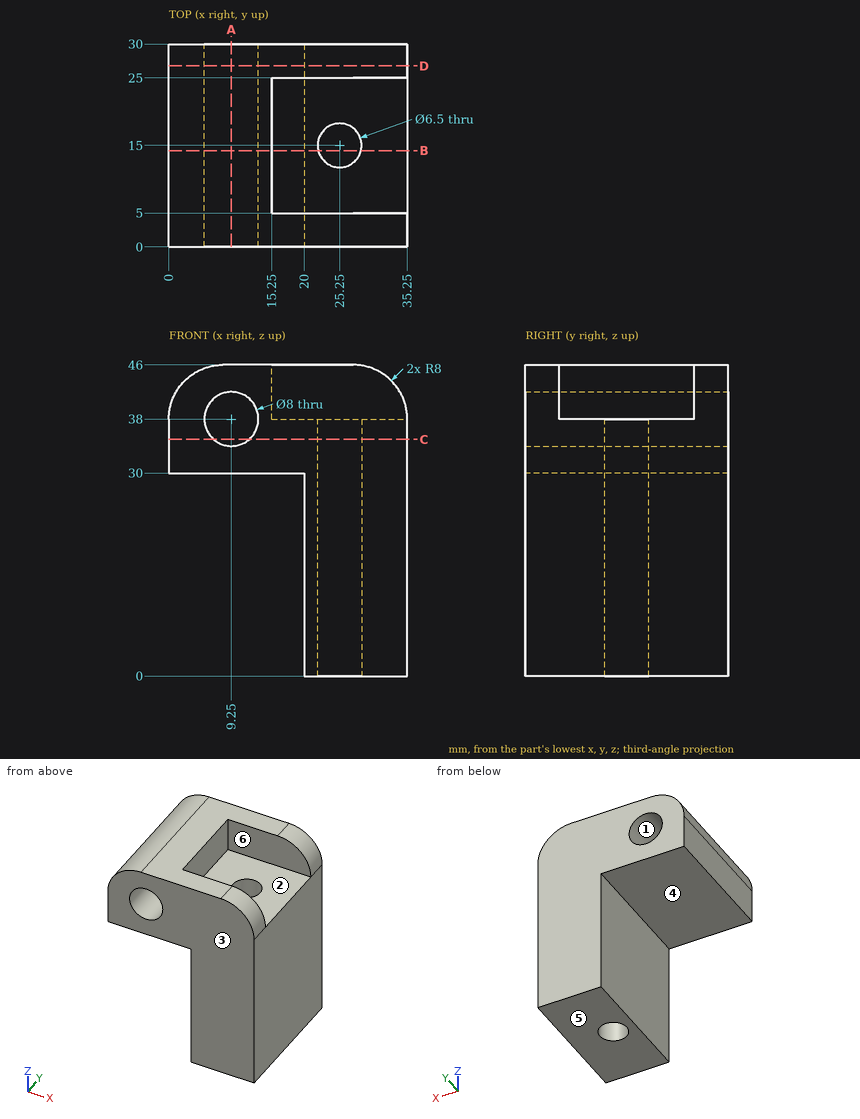
Verification items for this drawing (mm, ordinates from the low corner). A direction names the side the tool comes from. Coordinates: 2 decimals unless noted, no trailing zeros. Write each loop counter-clockwise with the first axis right and the second up, starting at its lowest first coordinate (ties: lowest second). Pieces come first, ordered by that corner, then holes. Notation, with made-up numbers: (35, 74) - (66, 74) arc R27 cw to (66, 90) - close; hole circle Ø4 at (12, -3.75). An arc over 180 degrees is marked (long way). One line per question, with ' | ' between items.
Item 1: Sectioned sample at B-B on y = 14.25. Record the boundary of the cut face in (x, z).
Determined:
outline: (0, 30) - (20, 30) - (20, 0) - (22.09, 0) - (22.09, 38) - (15.25, 38) - (15.25, 46) - (8, 46) arc R8 ccw to (0, 38) - close; (28.41, 0) - (35.25, 0) - (35.25, 38) - (28.41, 38) - close; hole circle Ø8 at (9.25, 38)
Item 2: Mould release check, pull along Y, two halves, no side actions. Record for the marked faces 1, 2 and 3: pulls with the +Y half, pulls with the -Y half, needs draft (parallel to the pull), parting line crosses it, or undercut.
Determined:
face 1: needs draft | face 2: undercut | face 3: pulls with the -Y half
Item 3: Gauge pin test, flat ends, axial feed: P1, Ø5, axis at x = 25.25, y = 15, coming from the -Z side; P2, Ø2, axis at x = 27.5, y = 15.5, coming from the +Z side; P3, Ø5, axis at y = 25.5, z = 18.5, coming from the -X side; P4, Ø6.5, axis at y = 11, z = 42, coming from the +X side. Record the tip position at first contact, or that the pin passes through.
Determined:
P1: passes through | P2: stops at z = 38 | P3: stops at x = 20 | P4: stops at x = 15.25
Item 4: Thickness scan on line 1 (Z direction, x = 9.25, y = 8.5); line 2 (Y direction, x = 25, z = 20); line 3 (X direction, y = 8.75, z = 28). Record the ranges inside material, lowest first. Write a range as [from, to].
Determined:
line 1: z = [30, 34], [42, 46] | line 2: y = [0, 11.76], [18.24, 30] | line 3: x = [20, 35.25]
Item 5: Sectioned sample at D-D on y = 26.75. Record the boundary of the cut face in (x, z).
Determined:
outline: (0, 30) - (20, 30) - (20, 0) - (35.25, 0) - (35.25, 38) arc R8 ccw to (27.25, 46) - (8, 46) arc R8 ccw to (0, 38) - close; hole circle Ø8 at (9.25, 38)
Item 6: Sectioned sample at C-C on z = 35. Record the boundary of the cut face in (x, y), plus the area to 3 significant figures.
Determined:
outline: (0, 0) - (6.6, 0) - (6.6, 30) - (0, 30) - close; (11.9, 0) - (35.25, 0) - (35.25, 30) - (11.9, 30) - close; hole circle Ø6.5 at (25.25, 15) | area: 866 mm2
Item 7: Sectioned sample at A-A on x = 9.25. Record the boundary of the cut face in (y, z).
Determined:
outline: (0, 30) - (30, 30) - (30, 34) - (0, 34) - close; (0, 42) - (30, 42) - (30, 46) - (0, 46) - close
Item 8: Access from +Z, -Z, +X, -X, +Y, -Y to the whole of each face (thin tool, end or side, straight path). Record for the marked faces 4, 5 and 6.
Determined:
face 4: -Z, -X, +Y, -Y | face 5: -Z, +X, -X, +Y, -Y | face 6: +Z, +X
